Input: part model. Units: mm. Frame: model coordinates. Face numbers are marked on the shaded views. Coordinates: 2 decimals unless noted, no trailing zeros. Write each loop counter-clockwise with the first axis right and the second up, starting at its lowest first coordinate (ties: lowest second). Pieces come first, ordered by that corner, then holes. Notation, with made-up numbers: M -39.75,42 L -7.75,42 A29 cw -7.75,64 Z; hole C 43,55.5 d9. An arc over 180 degrees is marked long. Use one line per item in the form item = value.
from build123d import *

# Parameters (mm, degrees)
SKETCH2_R           = 6.4
BOSS_EXTRUDE3_DEPTH = 3


with BuildPart() as part:
    # Sketch2 → Boss-Extrude3 (new body)
    with BuildSketch(Plane(origin=(0, 0, 0), x_dir=(0, 0, -1), z_dir=(1, 0, 0))):
        Polygon((-57.5, -15), (-79.5, -15), (-79.5, -5), (-82.5, -5), (-82.5, 5), (-79.5, 5), (-79.5, 15), (79.5, 15), (79.5, 5), (82.5, 5), (82.5, -5), (79.5, -5), (79.5, -15), (57.5, -15), (57.5, -18), (32.5, -18), (32.5, -15), (-32.5, -15), (-32.5, -18), (-57.5, -18), align=None)
        with Locations((0, 1)):
            Circle(SKETCH2_R, mode=Mode.SUBTRACT)
    extrude(amount=BOSS_EXTRUDE3_DEPTH)


solid = part.part
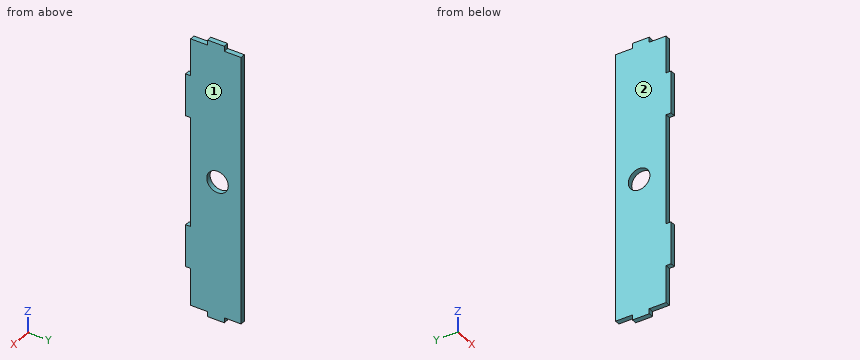
(1) Section query B-B on z = 0. Return the cut outline in (x, y).
Computed:
outline = M 0,-15 L 3,-15 L 3,-5.4 L 0,-5.4 Z; M 0,7.4 L 3,7.4 L 3,15 L 0,15 Z
(2) Section query A-A on y = 1. Return the cut outline in (x, z).
Computed:
outline = M 0,-82.5 L 3,-82.5 L 3,-6.4 L 0,-6.4 Z; M 0,6.4 L 3,6.4 L 3,82.5 L 0,82.5 Z
(3) First-contact query: pin 1 Ø0.9 at (x, y) = (2, 9.5) entering from +Z; pin 2 Ø1.5 at (x, z) = (1, -71) entering from -Y; pin 3 Ø0.9 at (x, y) = (1, -16) entering from +Z; pin 4 Ø3 at (y, z) = (-13.5, -2.5) entering from -X. Flat tips, straight axial feed; report the tip coordinate or a pass-through.
Computed:
pin_1 = 79.5
pin_2 = -15
pin_3 = 57.5
pin_4 = 0
(4) Pull-direction query (X, two-part tool) for the marked faces 1 and 2; classes: pulls with the +X half, pulls with the -X half, needs draft (parallel to the pull), parting line crosses it, or undercut.
Computed:
face_1 = pulls with the +X half
face_2 = pulls with the -X half
(5) Section query C-C on x = 1.65. Return the cut outline in (y, z), plus the area to 3 significant figures.
Computed:
outline = M -18,-57.5 L -15,-57.5 L -15,-79.5 L -5,-79.5 L -5,-82.5 L 5,-82.5 L 5,-79.5 L 15,-79.5 L 15,79.5 L 5,79.5 L 5,82.5 L -5,82.5 L -5,79.5 L -15,79.5 L -15,57.5 L -18,57.5 L -18,32.5 L -15,32.5 L -15,-32.5 L -18,-32.5 Z; hole C 1,0 d12.8
area = 4,850 mm^2
(6) Line query: probe 1 along Z at (x, y) = (1.1, -15.5); probe 2 along Y at (x, z) = (2, 0); probe 3 along Z at (x, y) = (2.6, -8.5). Output: solid intervals per line, ascending.
Computed:
probe_1 = -57.5 to -32.5, 32.5 to 57.5
probe_2 = -15 to -5.4, 7.4 to 15
probe_3 = -79.5 to 79.5
(7) Section query D-D on z = 69. Return the cut outline in (x, y), plus the area to 3 significant figures.
Computed:
outline = M 0,-15 L 3,-15 L 3,15 L 0,15 Z
area = 90.0 mm^2
